Part model, mm, in its own coordinate system. Face numbers are marked on the shaded views. A direction names the side the tool comes from. Give positions to 0.01 mm unless a question says otherwise; leave off trailing zeros. Write each loop counter-clockwise with the first axis right and the second up, starting at its lowest first coordinate (ties: lowest second). Pieces come first, ordered by that corner, then holes. Notation, with made-up numbers: M 77,79.25 L 91,79.25 A24 cw 91,99.25 Z; hole C 54,55 d3. An arc over 180 degrees is marked long. Use CSV: the item, a comma, the result in double quotes. Start each with the question number.
Item 1: Cut at D-D (y = 84). List the corners of the cut face in (x, z), then the cut area to 3 significant figures.
Item 2: Mould opens along Z. For the marked faces 3, 4, 5 and 6 say: released by +Z, released by -Z, zero draft, split by the parting line, or undercut.
Item 3: Cut at B-B (x = 96). List the corners of the cut face in (y, z).
Item 4: Drill centre lines: line 1 (Z direction, x = 51.5, y = 26); line 2 (X direction, y = 90, z = -89); line 3 (Y direction, x = 75, z = -87). Where is each one in solid material? Low to high. Write a range as [from, to].
Item 5: Cut at C-C (y = 196.5). List the corners of the cut face in (x, z), then the cut area to 3 significant figures.
Item 6: Cut at A-A (z = -30). List the corners of the cut face in (x, y), then the cut area to 3 significant figures.
Item 7: Pin check, flat tips, straight feed: pin 1 (5 mm diameter, centred on x = 120, z = -30, fed in from -Y); pin 2 (5 mm diameter, centred on x = 50, z = -52, fed in from -Y); pin 3 (4.5 mm diameter, centred on x = 120.31, y = 72.5, fed in from +Z); pin 4 (12 mm diameter, centred on x = 127.5, z = -22, fed in from -Y). Stop position of each tip, or through.
Item 8: Which spindle directions (+Z, -Z, +X, -X, +Y, -Y) get a long thin tool onto all of the face, cutting with end or side? Do the marked faces 1 and 2. Say none if no direction does.
from build123d import *

# Parameters (mm, degrees)
EXTRUDE_1_DEPTH          = 180
CUT_EXTRUDE_1_DEPTH      = 304.003530042
CUT_EXTRUDE_1_DEPTH_BACK = 304.003530042
SKETCH_14_R              = 30
SKETCH_14_R_2            = 2.75
CUT_EXTRUDE_3_DEPTH      = 50
SKETCH_15_R              = 27.5
EXTRUDE_3_DEPTH          = 10
SKETCH_16_R              = 17.5
SKETCH_16_R_2            = 2.25
CUT_EXTRUDE_4_DEPTH      = 32.5
SKETCH_17_R              = 2.75
CUT_EXTRUDE_5_DEPTH      = 6


with BuildPart() as part:
    # 草图11 → 拉伸-薄壁1 (new body)
    with BuildSketch(Plane(origin=(0, 0, 0), x_dir=(0, 0, -1), z_dir=(1, 0, 0))):
        Polygon((-84, 0), (-84, 180), (-50, 220.519622148), (50, 220.519622148), (84, 180), (84, 0), (90, 0), (90, 182.183821406), (52.797845949, 226.519622148), (-52.797845949, 226.519622148), (-90, 182.183821406), (-90, 0), align=None)
    extrude(amount=EXTRUDE_1_DEPTH)

    # 草图12 → 切除-拉伸1 (cut, two sides: drawn at the far end of the back side and taken through both)
    with BuildSketch(Plane.XY.offset(-CUT_EXTRUDE_1_DEPTH_BACK)):
        Polygon((0, 0), (0, 226.519622148), (45, 226.519622148), (30, 100), (30, 0), align=None)
        Polygon((150, 0), (180, 0), (180, 226.519622148), (135, 226.519622148), (150, 100), align=None)
    extrude(amount=CUT_EXTRUDE_1_DEPTH + CUT_EXTRUDE_1_DEPTH_BACK, mode=Mode.SUBTRACT)

    # 草图14 → 切除-拉伸3 (cut)
    with BuildSketch(Plane.XY.offset(90)):
        with Locations((90, 90)):
            Circle(SKETCH_14_R)
        with Locations((90, 125)):
            Circle(SKETCH_14_R_2)
        with Locations((107.5, 120.310889132)):
            Circle(SKETCH_14_R_2)
        with Locations((120.310889132, 107.5)):
            Circle(SKETCH_14_R_2)
        with Locations((125, 90)):
            Circle(SKETCH_14_R_2)
        with Locations((120.310889132, 72.5)):
            Circle(SKETCH_14_R_2)
        with Locations((107.5, 59.689110868)):
            Circle(SKETCH_14_R_2)
        with Locations((90, 55)):
            Circle(SKETCH_14_R_2)
        with Locations((72.5, 59.689110868)):
            Circle(SKETCH_14_R_2)
        with Locations((59.689110868, 72.5)):
            Circle(SKETCH_14_R_2)
        with Locations((55, 90)):
            Circle(SKETCH_14_R_2)
        with Locations((59.689110868, 107.5)):
            Circle(SKETCH_14_R_2)
        with Locations((72.5, 120.310889132)):
            Circle(SKETCH_14_R_2)
    extrude(amount=-CUT_EXTRUDE_3_DEPTH, mode=Mode.SUBTRACT)

    # 草图15 → 凸台-拉伸3 (add)
    with BuildSketch(Plane(origin=(0, 0, -90), x_dir=(-1, 0, 0), z_dir=(0, 0, -1))):
        with Locations(Location((-90, 90, 0), (0, 0, 270))):
            Circle(SKETCH_15_R)
    extrude(amount=EXTRUDE_3_DEPTH)

    # 草图16 → 切除-拉伸4 (cut)
    with BuildSketch(Plane(origin=(0, 0, -100), x_dir=(-1, 0, 0), z_dir=(0, 0, -1))):
        with Locations(Location((-90, 90, 0), (0, 0, 90))):
            Circle(SKETCH_16_R)
        with Locations(Location((-67.5, 90, 0), (0, 0, 90))):
            Circle(SKETCH_16_R_2)
        with Locations(Location((-74.090097423, 74.090097423, 0), (0, 0, 90))):
            Circle(SKETCH_16_R_2)
        with Locations(Location((-90, 67.5, 0), (0, 0, 90))):
            Circle(SKETCH_16_R_2)
        with Locations(Location((-105.909902577, 74.090097423, 0), (0, 0, 90))):
            Circle(SKETCH_16_R_2)
        with Locations(Location((-112.5, 90, 0), (0, 0, 90))):
            Circle(SKETCH_16_R_2)
        with Locations(Location((-105.909902577, 105.909902577, 0), (0, 0, 90))):
            Circle(SKETCH_16_R_2)
        with Locations(Location((-90, 112.5, 0), (0, 0, 90))):
            Circle(SKETCH_16_R_2)
        with Locations(Location((-74.090097423, 105.909902577, 0), (0, 0, 90))):
            Circle(SKETCH_16_R_2)
    extrude(amount=-CUT_EXTRUDE_4_DEPTH, mode=Mode.SUBTRACT)

    # 草图17 → 切除-拉伸5 (cut)
    with BuildSketch(Plane(origin=(0, 226.519622148, 0), x_dir=(1, 0, 0), z_dir=(0, 1, 0))):
        with Locations(Location((120, 30, 0), (0, 0, 270))):
            Circle(SKETCH_17_R)
        with Locations(Location((120, -30, 0), (0, 0, 90))):
            Circle(SKETCH_17_R)
        with Locations(Location((60, -30, 0), (0, 0, 270))):
            Circle(SKETCH_17_R)
        with Locations(Location((60, 30, 0), (0, 0, 90))):
            Circle(SKETCH_17_R)
    extrude(amount=-CUT_EXTRUDE_5_DEPTH, mode=Mode.SUBTRACT)


solid = part.part
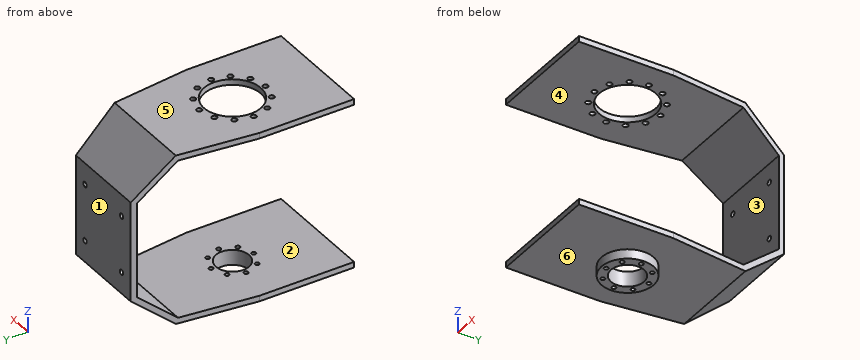
Worked answers:
1,outline,"M 30,-90 L 63.16,-90 L 63.16,-100 L 73.56,-100 L 73.56,-84 L 30,-84 Z; M 30,84 L 60.61,84 L 60.61,90 L 30,90 Z; M 106.44,-100 L 116.84,-100 L 116.84,-90 L 150,-90 L 150,-84 L 106.44,-84 Z; M 119.39,84 L 150,84 L 150,90 L 119.39,90 Z"
1,area,"1,100 mm^2"
2,face 3,"undercut"
2,face 4,"undercut"
2,face 5,"released by +Z"
2,face 6,"released by -Z"
3,outline,"M 0,-90 L 63.16,-90 L 63.16,-100 L 73.56,-100 L 73.56,-84 L 0,-84 Z; M 0,84 L 60.61,84 L 60.61,90 L 0,90 Z; M 106.44,-100 L 116.84,-100 L 116.84,-90 L 182.18,-90 L 226.52,-52.8 L 226.52,52.8 L 182.18,90 L 119.39,90 L 119.39,84 L 180,84 L 220.52,50 L 220.52,-50 L 180,-84 L 106.44,-84 Z"
4,line 1,"z = [-90, -84], [84, 90]"
4,line 2,"x = [30, 65.25], [69.75, 72.5], [107.5, 110.25], [114.75, 150]"
4,line 3,"y = [0, 72.03], [76.15, 80.99], [99.01, 103.85], [107.97, 185.76]"
5,outline,"M 41.44,-77.99 L 138.56,-77.99 L 138.56,-70.15 L 41.44,-70.15 Z; M 41.44,70.15 L 138.56,70.15 L 138.56,77.99 L 41.44,77.99 Z"
5,area,"1,520 mm^2"
6,outline,"M 44.29,220.52 L 57.25,220.52 L 57.25,226.52 L 45,226.52 Z; M 62.75,220.52 L 117.25,220.52 L 117.25,226.52 L 62.75,226.52 Z; M 122.75,220.52 L 135.71,220.52 L 135,226.52 L 122.75,226.52 Z"
6,area,"478 mm^2"
7,pin 1,"passes through"
7,pin 2,"stops at y = 215.16"
7,pin 3,"stops at z = -84"
7,pin 4,"stops at y = 220.52"
8,face 1,"+Z, -Z, +X, -X, +Y"
8,face 2,"+X, -X, -Y"
